CAD build for the part. Positions are in the model's coordinates, mm. Face numbers are marked on the shaded views. A direction names the side the tool comes from. Give positions to 0.01 mm unless a question says otherwise; leave off trailing zeros. Order: outer loops, then holes, each group sorted by start corner. A loop starts at its lowest first (then second) coordinate and runs counter-clockwise, first axis right, second up.
from build123d import *

# Parameters (mm, degrees)
BOSS_EXTRUDE1_DEPTH      = 18.25
BOSS_EXTRUDE1_DEPTH_BACK = 18.25
SKETCH4_R                = 4.2
CUT_EXTRUDE1_DEPTH       = 6
SKETCH6_R                = 10
CUT_EXTRUDE2_DEPTH       = 35


with BuildPart() as part:
    # Sketch2 → Boss-Extrude1 (new body, two sides)
    with BuildSketch(Plane.XY) as boss_extrude1_sk:
        Polygon((-20, 20), (-20, -20), (20, -20), (20, -14), (-14, 20), align=None)
        Polygon((-14, 11.514718626), (-14, -14), (11.514718626, -14), align=None, mode=Mode.SUBTRACT)
    extrude(amount=BOSS_EXTRUDE1_DEPTH)
    extrude(boss_extrude1_sk.sketch, amount=-BOSS_EXTRUDE1_DEPTH_BACK)

    # Sketch4 → Cut-Extrude1 (cut)
    with BuildSketch(Plane.XZ.offset(20)):
        Circle(SKETCH4_R)
    cut_extrude1 = extrude(amount=-CUT_EXTRUDE1_DEPTH, mode=Mode.SUBTRACT)

    # Sketch6 → Cut-Extrude2 (cut, through all)
    with BuildSketch(Plane(origin=(0, -14, 0), x_dir=(1, 0, 0), z_dir=(0, 1, 0))):
        Circle(SKETCH6_R)
    cut_extrude2 = extrude(amount=CUT_EXTRUDE2_DEPTH, mode=Mode.SUBTRACT)

    # Mirror1: Cut-Extrude1, Cut-Extrude2 across plane
    add(cut_extrude1.mirror(Plane(origin=(0, 0, 0), x_dir=(0, 0, 1), z_dir=(0.707106781, -0.707106781, 0))), mode=Mode.SUBTRACT)
    add(cut_extrude2.mirror(Plane(origin=(0, 0, 0), x_dir=(0, 0, 1), z_dir=(0.707106781, -0.707106781, 0))), mode=Mode.SUBTRACT)


solid = part.part
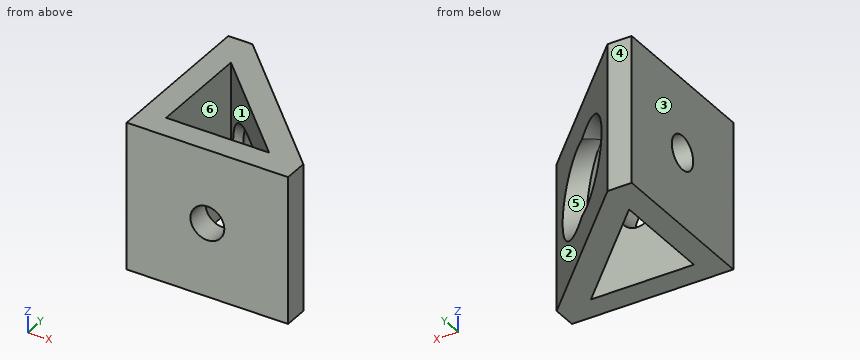
1. Saw through at D-D on y = 1. Give the cut face in (x, z).
2. Wall check: line 1 (Z direction, x = -17, y = 0); line 2 (Y direction, x = 9.5, z = 1.5). Give the ranges that are in metal, low to high.
3. Saw through at A-A on z = 0. Give the cut face in (x, y), plus the area to 3 significant figures.
4. Saw through at C-C on y = 9. Give the cut face in (x, z).
5. 3-axis set-ups, long thin cutter, end or side, ignore diameter. For the marked faces 4, 5 and 6: which of +Z, -Z, +X, -X, +Y, -Y reach the whole face in a straight line?
6. Mould opens along X. For the marked faces 1, 2 and 3 say: released by +X, released by -X, zero draft, split by the parting line, or undercut.
7. Saw through at B-B on z = 15. Give the cut face in (x, y).
8. Pin check, flat tips, straight feed: P1, Ø11, axis at x = 0, z = 0, coming from the +Y side; P2, Ø16, axis at y = 0, z = 0, coming from the -X side; P3, Ø4, axis at x = 9.5, z = 11.5, coming from the +Y side; P4, Ø7.5, axis at y = 3.5, z = 7.5, coming from the +X side. Stop position of each tip, or through.
Reported:
1. outline: (-20, -18.25) - (-14, -18.25) - (-14, -4.08) - (-20, -4.08) - close; (-20, 4.08) - (-14, 4.08) - (-14, 18.25) - (-20, 18.25) - close; (-3.49, -18.25) - (5, -18.25) - (5, -9.95) - (1, -9.95) arc R10 cw to (-1, -9.95) - (-3.49, -9.95) - close; (-3.49, 9.95) - (-1, 9.95) arc R10 cw to (1, 9.95) - (5, 9.95) - (5, 18.25) - (-3.49, 18.25) - close
2. line 1: z = -18.25 to -4.2, 4.2 to 18.25
2. line 2: y = -20 to -14
3. outline: (-20, -20) - (-4.2, -20) - (-4.2, -14) - (-14, -14) - (-14, -4.2) - (-20, -4.2) - close; (-20, 4.2) - (-14, 4.2) - (-14, 11.51) - (-12.49, 10) - (-10, 10) - (-10, 16) - (-14, 20) - (-20, 20) - close; (4.2, -20) - (20, -20) - (20, -14) - (16, -10) - (10, -10) - (10, -12.49) - (11.51, -14) - (4.2, -14) - close
3. area: 405 mm2
4. outline: (-20, -18.25) - (-14, -18.25) - (-14, 18.25) - (-20, 18.25) - close; (-11.49, -18.25) - (-3, -18.25) - (-3, -9.54) arc R10 cw to (-9, -4.36) - (-11.49, -4.36) - close; (-11.49, 4.36) - (-9, 4.36) arc R10 cw to (-3, 9.54) - (-3, 18.25) - (-11.49, 18.25) - close
5. face 4: +Z, -Z, +X, -X, +Y
5. face 5: +X
5. face 6: +Z, -Z
6. face 1: undercut
6. face 2: released by +X
6. face 3: released by -X
7. outline: (-20, -20) - (20, -20) - (20, -14) - (-14, 20) - (-20, 20) - close; hole (-14, -14) - (11.51, -14) - (-14, 11.51) - close
8. P1: stops at y = -14
8. P2: stops at x = -20
8. P3: stops at y = -1.5
8. P4: stops at x = 5.32
